Geometry: final body of the model. Coordinates: model frame, mm. Face numbers are marked on the shaded views. A direction names the side the tool comes from. Give positions to 0.01 mm unless a question says otherwise; leave off trailing zeros. Write each loop counter-clockwise with the first axis right and the second up, starting at its lowest first coordinate (ties: lowest second). Pieces come first, ordered by that corner, then holes.
```python
from build123d import *

# Parameters (mm, degrees)
SKETCH_9_OUTSIDE_W     = 66.002
SKETCH_9_OUTSIDE_H     = 66.002
SKETCH_9_OUTSIDE_R     = 1.5
SKETCH_9_OUTSIDE_R_2   = 3
CUT_EXTRUDE_2_DEPTH    = 63.557973113
HOLE_WIZARD_M3_1_D     = 2.5
HOLE_WIZARD_M3_1_DEPTH = 7.5
HOLE_WIZARD_M3_1_TIP   = 0.751075774
SKETCH_10_R            = 4
CUT_EXTRUDE_3_DEPTH    = 62.601489889
SKETCH_15_R            = 6
CUT_EXTRUDE_4_DEPTH    = 40
CHAMFER_1_SIZE         = 2


with BuildPart() as part:
    # 草图2 → 旋转1 (revolve)
    with BuildSketch(Plane.XY, mode=Mode.PRIVATE) as revolve_1_sk:
        Polygon((0, 0), (23.5, 0), (23.5, 2.5), (9, 2.5), (9, 53), (0, 53), align=None)
    revolve(revolve_1_sk.sketch.rotate(Axis((0, 0, 0), (0, 1, 0)), 90), axis=Axis((0, 0, 0), (0, 1, 0)))

    # 草图9 outside → 切除-拉伸2 (cut, through all)
    # profile 1 of 7: a face of its own
    with BuildSketch(Plane.XZ):
        Rectangle(SKETCH_9_OUTSIDE_W, SKETCH_9_OUTSIDE_H)
        with BuildLine():
            Line((-3.031088913, 21.75), (-20.351596989, -8.25))
            ThreePointArc((-20.351596989, -8.25), (-20.351596989, -11.75), (-17.320508076, -13.5))
            Line((-17.320508076, -13.5), (17.320508076, -13.5))
            ThreePointArc((17.320508076, -13.5), (20.351596989, -11.75), (20.351596989, -8.25))
            Line((20.351596989, -8.25), (3.031088913, 21.75))
            ThreePointArc((3.031088913, 21.75), (0, 23.5), (-3.031088913, 21.75))
        make_face(mode=Mode.SUBTRACT)
    # profile 2 of 7: a face of its own
    with BuildSketch(Plane.XZ):
        with Locations(Location((0, 20, 0), (0, 0, 270))):
            Circle(SKETCH_9_OUTSIDE_R)
    # profile 3 of 7: a face of its own
    with BuildSketch(Plane.XZ):
        with Locations(Location((17.320508076, -10, 0), (0, 0, 270))):
            Circle(SKETCH_9_OUTSIDE_R)
    # profile 4 of 7: a face of its own
    with BuildSketch(Plane.XZ):
        with Locations(Location((-17.320508076, -10, 0), (0, 0, 270))):
            Circle(SKETCH_9_OUTSIDE_R)
    # profile 5 of 7: a face of its own
    with BuildSketch(Plane.XZ):
        with Locations(Location((0, 13, 0), (0, 0, 270))):
            Circle(SKETCH_9_OUTSIDE_R_2)
    # profile 6 of 7: a face of its own
    with BuildSketch(Plane.XZ):
        with Locations(Location((11.258330249, -6.5, 0), (0, 0, 270))):
            Circle(SKETCH_9_OUTSIDE_R_2)
    # profile 7 of 7: a face of its own
    with BuildSketch(Plane.XZ):
        with Locations(Location((-11.258330249, -6.5, 0), (0, 0, 270))):
            Circle(SKETCH_9_OUTSIDE_R_2)
    extrude(amount=-CUT_EXTRUDE_2_DEPTH, mode=Mode.SUBTRACT)

    # M3 螺纹孔1
    with Locations(Plane(origin=(0, 53, 0), x_dir=(1, 0, 0), z_dir=(0, 1, 0))):
        with Locations((-5.629165125, -3.25), (0, 6.5), (5.629165125, -3.25)):
            Hole(HOLE_WIZARD_M3_1_D / 2, depth=HOLE_WIZARD_M3_1_DEPTH)
            with Locations((0, 0, -(HOLE_WIZARD_M3_1_DEPTH + HOLE_WIZARD_M3_1_TIP / 2))):  # 118° drill point
                Cone(0, HOLE_WIZARD_M3_1_D / 2, HOLE_WIZARD_M3_1_TIP, mode=Mode.SUBTRACT)

    # 草图10 → 切除-拉伸3 (cut, through all)
    with BuildSketch(Plane(origin=(0, 53, 0), x_dir=(1, 0, 0), z_dir=(0, 1, 0))):
        with Locations(Location((0, 0, 0), (0, 0, 270))):
            Circle(SKETCH_10_R)
    extrude(amount=-CUT_EXTRUDE_3_DEPTH, mode=Mode.SUBTRACT)

    # 草图15 → 切除-拉伸4 (cut)
    with BuildSketch(Plane.XZ):
        with Locations(Location((0, 0, 0), (0, 0, 270))):
            Circle(SKETCH_15_R)
    extrude(amount=-CUT_EXTRUDE_4_DEPTH, mode=Mode.SUBTRACT)

    # 倒角1
    chamfer_1_edges = [part.edges().sort_by_distance(p)[0] for p in [
        (0, 40, 6),
    ]]
    chamfer(chamfer_1_edges, length=CHAMFER_1_SIZE - 0.0001)  # a hair under: the kernel refuses the full size


solid = part.part
```
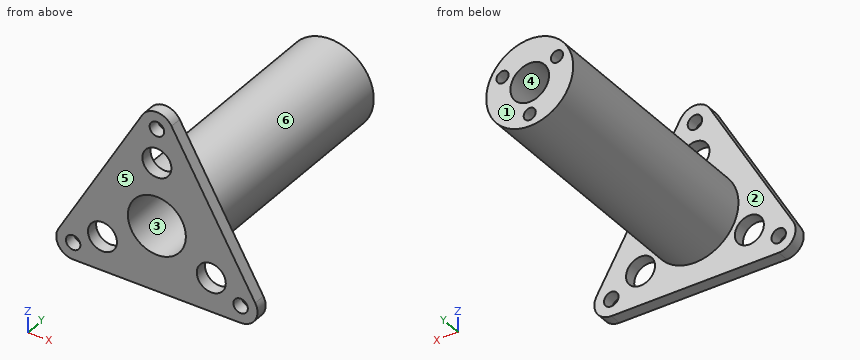
Item 1: Section C-C, the plane z = 12.5. Return the cut outline in (x, y), plus the area to 3 significant figures.
Found:
outline: (-8.37, 0) - (-2.96, 0) - (-2.96, 2.5) - (-8.37, 2.5) - close; (2.96, 0) - (8.37, 0) - (8.37, 2.5) - (2.96, 2.5) - close
area: 27.1 mm2
Item 2: Section B-B, the plane y = 8. Return the cut outline in (x, z), plus the area to 3 significant figures.
Found:
outline: circle Ø18 at (0, 0); hole circle Ø12 at (0, 0)
area: 141 mm2
Item 3: Line query: L1, parallel to X at y = 26.5, z = 0; L2, parallel to X at y = 1.9, z = -6.5; L3, parallel to X at y = 48, z = 0. Output: solid intervals per line, ascending.
Found:
L1: x = -9 to -6, 6 to 9
L2: x = -19.34 to -14.26, -8.26 to 8.26, 14.26 to 19.34
L3: x = -9 to -4, 4 to 9
Item 4: Pin query (flat end, axial travel): pin 1 Ø5 at (x, z) = (0.5, -5.5) entering from -Y; pin 2 Ø6 at (x, y) = (-7, 19.5) entering from -Z; pin 3 Ø7 at (x, z) = (11.26, -6.5) entering from +Y; pin 4 Ø2 at (x, y) = (7, 31) entering from +Z. Return the tip coordinate at first contact, or that it passes through.
Found:
pin 1: stops at y = 0
pin 2: stops at z = -8.06
pin 3: stops at y = 2.5
pin 4: stops at z = 6.71
Item 5: Section D-D, the plane y = 42. Return the cut outline in (x, z), plus the area to 3 significant figures.
Found:
outline: circle Ø18 at (0, 0); hole circle Ø8 at (0, 0)
area: 204 mm2
Item 6: Pull-direction query (Z, two-part tool) for the marked faces 4, 5 and 6; classes: +Z half, -Z half, draft (parallel to the pull), parting line (faces both ways), or undercut.
Found:
face 4: undercut
face 5: draft
face 6: parting line
Item 7: Reachability of the marked faces 1, 2 and 3 from +Z, -Z, +X, -X, +Y, -Y: full face, straight path, thin tool, end or side. Return the list, or none.
Found:
face 1: +Z, -Z, +X, -X, +Y
face 2: +Y
face 3: -Y
